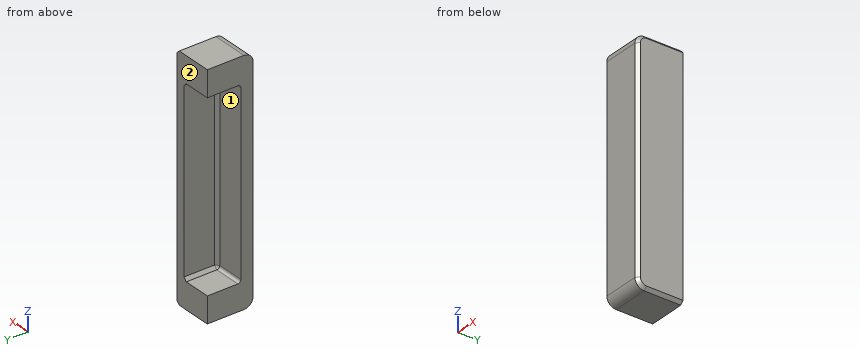
Autodesk Fusion 360 part; units mm, degrees
sketch "Sketch1" plane through (0, 0, 0) normal (1, 0, 0) x (0, 1, 0)
  line L0 (0, 0) -> (-12, 0)
  arc A0 (-15, 3) -> (-12, 0) centre (-12, 3) ccw
  line L1 (-15, 3) -> (-15, 74)
  arc A1 (-12, 77) -> (-15, 74) centre (-12, 74) ccw
  line L2 (-12, 77) -> (0, 77)
  line L3 (0, 77) -> (0, 0)
  line L4 (0, 68.5) -> (-11, 68.5)
  line L5 (-11, 68.5) -> (-11, 8.5)
  line L6 (-11, 8.5) -> (0, 8.5)
  line L7 (-11, 38.5) -> (-15, 38.5) construction
  dimension "d1" = 60
  dimension "d2" = 77
  dimension "d3" = 3
  dimension "d4" = 15
  dimension "d5" = 11
extrude "Extrude1" add sketch "Sketch1" against normal blind 10 contours L0 A0 L1 A1 L2 L3 L4 L5 L6
extrude "Extrude2" add sketch "Sketch1" along normal blind 3
fillet "Fillet1" radius 1 2 edges at (-5, -11, 68.5) (-5, -11, 8.5)
chamfer "Chamfer1" distance 1 angle 45 10 edges at (3, -6, 77) (3, -14.1213, 76.1213) (3, -15, 38.5) (3, -14.1213, 0.8787) (3, -6, 0) (0, -5, 68.5) (0, -10.7071, 68.2071) (0, -11, 38.5) (0, -10.7071, 8.7929) (0, -5, 8.5)
Work out the finished part from the listing and answer in its coordinate system (mm). Face numbers are marked on the shaded views. A direction names the side the tool comes from. Give positions to 0.01 mm unless a question says otherwise; leave off trailing zeros. Order: outer loops, then holes, each group sorted by start corner. A loop starts at its lowest first (then second) coordinate and runs counter-clockwise, first axis right, second up. Notation, with made-up numbers: (46.5, 24.25) -> (61.5, 24.25) arc R25 ccw to (61.5, 53.25) -> close; hole circle Ø10 at (30.5, -20.75). An arc over 180 degrees is marked (long way). One line per item, written item: value.
Item 1: Find section C-C, the plane x = -7.75. Give the vertices of the cut face in (y, z), plus the area to 3 significant figures.
Answer sheet:
outline: (-15, 3) arc R3 ccw to (-12, 0) -> (0, 0) -> (0, 8.5) -> (-10, 8.5) arc R1 cw to (-11, 9.5) -> (-11, 67.5) arc R1 cw to (-10, 68.5) -> (0, 68.5) -> (0, 77) -> (-12, 77) arc R3 ccw to (-15, 74) -> close
area: 492 mm²
Item 2: Straight lines are drawn through the part: probe 1 along Z at (x, y) = (-2.5, -9); probe 2 along X at (y, z) = (-1, 19.5); probe 3 along Y at (x, z) = (-6.75, 9.5). For each, find the intervals that lie inside material, in ascending order.
Answer sheet:
probe 1: 0 to 8.5, 68.5 to 77
probe 2: 0 to 3
probe 3: -15 to -11
Item 3: Find section B-B, the plane y = -4.75. Give the vertices of the cut face in (x, z).
Answer sheet:
outline: (-10, 0) -> (2, 0) -> (3, 1) -> (3, 76) -> (2, 77) -> (-10, 77) -> (-10, 68.5) -> (-1, 68.5) -> (0, 67.5) -> (0, 9.5) -> (-1, 8.5) -> (-10, 8.5) -> close
Item 4: Find section A-A, the plane z = 55.5. Give the vertices of the cut face in (x, y).
Answer sheet:
outline: (-10, -15) -> (2, -15) -> (3, -14) -> (3, 0) -> (0, 0) -> (0, -10) -> (-1, -11) -> (-10, -11) -> close
Item 5: Flat-ended cylindrical pins translate along their axes: P1, Ø5, axis at y = -4, z = 36, coming from the -X side; P2, Ø3, axis at y = -9, z = 49.5, coming from the -X side; P3, Ø2, axis at x = -3.5, z = 66, coming from the +Y side. Find the tip coordinate at first contact, or state that the pin passes through.
Answer sheet:
P1: x = 0
P2: x = -0.5
P3: y = -11
Item 6: A tool of negligible diameter and unlimited length cuts with its end or side. For the marked faces 1 and 2, from which of +Z, -Z, +X, -X, +Y, -Y can it reach the whole face along a straight path? Write none if from no direction.
Answer sheet:
face 1: -X, +Y
face 2: +Z, -Z, +X, -X, +Y
